Model file for the job. Use its own axes, mm. Face numbers are marked on the shaded views. A direction names the side the tool comes from. Round coordinates to 2 decimals unless told otherwise and drop trailing zeros. Order: outer loops, then holes, each group sorted by start corner. A loop starts at its lowest first (then second) coordinate and runs counter-clockwise, first axis right, second up. Notation, with made-up numbers: (72, 52) -> (108, 52) arc R23 cw to (108, 90) -> close; hole circle Ø6 at (74, 41). An arc over 180 degrees is marked (long way). Put each result on its own line as item: value. Start each with the question number.
Q1. Cut at C-C, the plane z = 61. List the corners of the cut face in (x, y).
Q2. Cut at B-B, the plane x = 74. List the corners of the cut face in (y, z).
Q3. Cut at D-D, the plane y = 18.75. List the corners of the cut face in (x, z).
Q4. Probe L1, parallel to Z at x = 73, y = 8.75; L2, parallel to Y at x = 71.5, z = 54; L3, parallel to X at y = 7.75, z = 83. List the from-to ranges inside material, lowest first.
Q5. Pull direction Y, two halves, no side cores. Call the marked faces 1, 2 and 3: released by +Y, released by -Y, zero draft, split by the parting line, or undercut.
Q6. Cut at A-A, the plane y = 4. List the corners of the cut face in (x, z).
Q7. Flat gauge pins, fed straight in: P1, Ø6.5, axis at x = 73, y = 16, coming from the +Z side; P2, Ø2.5, axis at y = 12.5, z = 83, coming from the -X side; P3, Ø4, axis at y = 13, z = 83.5, coming from the +X side; P4, Ø10.5, axis at x = 52, y = 12, coming from the +Z side. Where does each tip first touch, or does it go through?
Q8. 3-axis set-ups, long thin cutter, end or side, ignore diameter. For the marked faces 4, 5 and 6: which of +Z, -Z, +X, -X, +Y, -Y reach the whole face in a straight line?
Autodesk Fusion 360 part; units mm, degrees
sketch "Sketch1" plane through (0, 0, 0) normal (0, 1, 0) x (1, 0, 0)
  line L0 (5.08, -7.62) -> (93.98, -7.62)
  line L1 (93.98, -7.62) -> (93.98, -96.52)
  line L2 (93.98, -96.52) -> (5.08, -96.52)
  line L3 (5.08, -96.52) -> (5.08, -7.62)
  dimension "d1" = 88.9
  dimension "d2" = 88.9
extrude "Extrude1" add sketch "Sketch1" along normal blind 2.54
sketch "Sketch2" plane through (0, 2.54, 0) normal (0, 1, 0) x (-1, 0, 0)
  line L0 (-5.08, 96.52) -> (-93.98, 96.52)
  line L1 (-93.98, 96.52) -> (-93.98, 7.62)
  line L2 (-93.98, 7.62) -> (-5.08, 7.62)
  line L3 (-5.08, 7.62) -> (-5.08, 96.52)
  line L4 (-17.78, 20.32) -> (-81.28, 20.32)
  line L5 (-81.28, 20.32) -> (-81.28, 83.82)
  line L6 (-81.28, 83.82) -> (-17.78, 83.82)
  line L7 (-17.78, 83.82) -> (-17.78, 20.32)
  dimension "d5" = 63.5
  dimension "d6" = 63.5
  dimension "d7" = 12.7
  dimension "d8" = 12.7
extrude "Extrude2" add sketch "Sketch2" along normal blind 2.54 contours L4 L5 L6 L7
sketch "Sketch3" plane through (0, 5.08, 0) normal (0, 1, 0) x (-1, 0, 0)
  line L0 (-17.78, 83.82) -> (-81.28, 83.82)
  line L1 (-81.28, 83.82) -> (-81.28, 20.32)
  line L2 (-81.28, 20.32) -> (-17.78, 20.32)
  line L3 (-17.78, 20.32) -> (-17.78, 83.82)
  line L4 (-17.78, 20.32) -> (-30.48, 20.32)
  line L5 (-30.48, 20.32) -> (-30.48, 22.86)
  line L6 (-30.48, 22.86) -> (-17.78, 22.86)
  line L7 (-17.78, 22.86) -> (-17.78, 20.32)
  line L8 (-81.28, 20.32) -> (-68.58, 20.32)
  line L9 (-68.58, 20.32) -> (-68.58, 22.86)
  line L10 (-68.58, 22.86) -> (-81.28, 22.86)
  line L11 (-81.28, 22.86) -> (-81.28, 20.32)
  line L12 (-17.78, 83.82) -> (-30.48, 83.82)
  line L13 (-30.48, 83.82) -> (-30.48, 81.28)
  line L14 (-30.48, 81.28) -> (-17.78, 81.28)
  line L15 (-17.78, 81.28) -> (-17.78, 83.82)
  line L16 (-81.28, 83.82) -> (-68.58, 83.82)
  line L17 (-68.58, 83.82) -> (-68.58, 81.28)
  line L18 (-68.58, 81.28) -> (-81.28, 81.28)
  line L19 (-81.28, 81.28) -> (-81.28, 83.82)
extrude "Extrude3" add sketch "Sketch3" along normal blind 10.31 contours L0 L3 L12 L13 L14 L15 | L0 L1 L16 L17 L18 L19 | L2 L3 L4 L5 L6 L7 | L1 L2 L8 L9 L10 L11
sketch "Sketch4" plane through (0, 15.39, 0) normal (0, 1, 0) x (-1, 0, 0)
  line L0 (-81.28, 81.28) -> (-68.58, 81.28)
  line L1 (-68.58, 81.28) -> (-68.58, 83.82)
  line L2 (-68.58, 83.82) -> (-81.28, 83.82)
  line L3 (-81.28, 83.82) -> (-81.28, 81.28)
  line L4 (-30.48, 81.28) -> (-17.78, 81.28)
  line L5 (-17.78, 81.28) -> (-17.78, 86.36)
  line L6 (-17.78, 86.36) -> (-30.48, 86.36)
  line L7 (-30.48, 86.36) -> (-30.48, 81.28)
  line L8 (-17.78, 22.86) -> (-30.48, 22.86)
  line L9 (-30.48, 22.86) -> (-30.48, 17.78)
  line L10 (-30.48, 17.78) -> (-17.78, 17.78)
  line L11 (-17.78, 17.78) -> (-17.78, 22.86)
  line L12 (-68.58, 22.86) -> (-81.28, 22.86)
  line L13 (-81.28, 22.86) -> (-81.28, 17.78)
  line L14 (-81.28, 17.78) -> (-68.58, 17.78)
  line L15 (-68.58, 17.78) -> (-68.58, 22.86)
  line L16 (-81.28, 81.28) -> (-68.58, 81.28)
  line L17 (-68.58, 81.28) -> (-68.58, 86.36)
  line L18 (-68.58, 86.36) -> (-81.28, 86.36)
  line L19 (-81.28, 86.36) -> (-81.28, 81.28)
  dimension "d17" = 5.08
  dimension "d18" = 5.08
  dimension "d19" = 5.08
  dimension "d20" = 5.08
extrude "Extrude4" add sketch "Sketch4" along normal blind 6.35
sketch "Sketch5" plane through (81.28, 0, 0) normal (1, 0, 0) x (0, 0, -1)
  line L0 (-83.82, 2.54) -> (-20.32, 2.54)
  line L1 (-20.32, 2.54) -> (-20.32, 15.39)
  line L2 (-20.32, 15.39) -> (-17.78, 15.39)
  line L3 (-17.78, 15.39) -> (-17.78, 21.74)
  line L4 (-17.78, 21.74) -> (-22.86, 21.74)
  line L5 (-22.86, 21.74) -> (-22.86, 5.08)
  line L6 (-22.86, 5.08) -> (-81.28, 5.08)
  line L7 (-81.28, 5.08) -> (-81.28, 21.74)
  line L8 (-81.28, 21.74) -> (-86.36, 21.74)
  line L9 (-86.36, 21.74) -> (-86.36, 15.39)
  line L10 (-86.36, 15.39) -> (-83.82, 15.39)
  line L11 (-83.82, 15.39) -> (-83.82, 2.54)
  line L12 (-86.36, 15.39) -> (-81.28, 21.74)
  line L13 (-86.36, 21.74) -> (-86.36, 15.39)
  line L14 (-81.28, 21.74) -> (-86.36, 21.74)
  line L15 (-22.86, 21.74) -> (-17.78, 15.39)
  line L16 (-17.78, 21.74) -> (-22.86, 21.74)
extrude "Extrude5" cut sketch "Sketch5" against normal blind 63.5 contours L8 L9 L12 L13 L14 | L3 L4 L15 L16
sketch "Sketch6" plane through (0, 5.08, 0) normal (0, 1, 0) x (-1, 0, 0)
  line L0 (-30.48, 81.28) -> (-30.48, 83.82)
  line L1 (-30.48, 83.82) -> (-68.58, 83.82)
  line L2 (-68.58, 83.82) -> (-68.58, 81.28)
  line L3 (-68.58, 81.28) -> (-81.28, 81.28)
  line L4 (-81.28, 81.28) -> (-81.28, 22.86)
  line L5 (-81.28, 22.86) -> (-68.58, 22.86)
  line L6 (-68.58, 22.86) -> (-68.58, 20.32)
  line L7 (-68.58, 20.32) -> (-30.48, 20.32)
  line L8 (-30.48, 20.32) -> (-30.48, 22.86)
  line L9 (-30.48, 22.86) -> (-17.78, 22.86)
  line L10 (-17.78, 22.86) -> (-17.78, 81.28)
  line L11 (-17.78, 81.28) -> (-30.48, 81.28)
  line L12 (-22.86, 78.74) -> (-76.2, 78.74)
  line L13 (-76.2, 78.74) -> (-76.2, 25.4)
  line L14 (-76.2, 25.4) -> (-22.86, 25.4)
  line L15 (-22.86, 25.4) -> (-22.86, 78.74)
extrude "Extrude6" cut sketch "Sketch6" against normal blind 2.54 contours L12 L13 L14 L15
equation "d11 = 0.4 in + 0.15 mm"
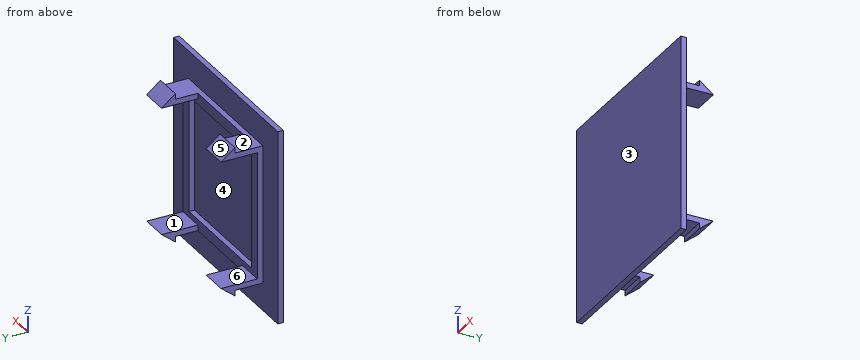
Ans:
1. outline: (5.08, 0) -> (93.98, 0) -> (93.98, 2.54) -> (81.28, 2.54) -> (81.28, 5.08) -> (76.2, 5.08) -> (76.2, 2.54) -> (22.86, 2.54) -> (22.86, 5.08) -> (17.78, 5.08) -> (17.78, 2.54) -> (5.08, 2.54) -> close
2. outline: (0, 7.62) -> (2.54, 7.62) -> (2.54, 20.32) -> (15.39, 20.32) -> (15.39, 17.78) -> (21.74, 22.86) -> (5.08, 22.86) -> (5.08, 25.4) -> (2.54, 25.4) -> (2.54, 78.74) -> (5.08, 78.74) -> (5.08, 81.28) -> (21.74, 81.28) -> (15.39, 86.36) -> (15.39, 83.82) -> (2.54, 83.82) -> (2.54, 96.52) -> (0, 96.52) -> close
3. outline: (17.78, 20.47) -> (30.48, 20.47) -> (30.48, 22.86) -> (17.78, 22.86) -> close; (17.78, 81.28) -> (30.48, 81.28) -> (30.48, 83.67) -> (17.78, 83.67) -> close; (68.58, 20.47) -> (81.28, 20.47) -> (81.28, 22.86) -> (68.58, 22.86) -> close; (68.58, 81.28) -> (81.28, 81.28) -> (81.28, 83.67) -> (68.58, 83.67) -> close
4. L1: z = 20.32 to 22.86, 81.28 to 83.82
4. L2: y = 0 to 2.54
4. L3: x = 17.78 to 30.48, 68.58 to 81.28
5. face 1: zero draft
5. face 2: undercut
5. face 3: released by -Y
6. outline: (17.78, 20.32) -> (81.28, 20.32) -> (81.28, 83.82) -> (17.78, 83.82) -> close; hole (22.86, 25.4) -> (76.2, 25.4) -> (76.2, 78.74) -> (22.86, 78.74) -> close
7. P1: stops at z = 86.36
7. P2: stops at x = 17.78
7. P3: stops at x = 81.28
7. P4: passes through
8. face 4: +Y
8. face 5: +Z, +X, -X, +Y
8. face 6: +X, -X, +Y
